Part model, mm, in its own coordinate system. A direction names the side the tool comes from. Round coordinates to 2 decimals unless told otherwise and drop trailing zeros. Loops run counter-clockwise (first coordinate to the right, second up) from the corner with the lowest first, then second, coordinate; pieces in that order, holes last. Notation, with made-up numbers: M -21.5,45 L 30.5,45 A23 ccw 30.5,63 Z; hole C -5.75,6 d2. An arc over 180 degrees is marked long. Answer as CSV lines item,"result". Start each with the question number.
Item 1: Wall check: line 1 (Y direction, x = 25.85, z = 1); line 2 (X direction, y = 2, z = 0.5); line 3 (X direction, y = 3, z = 1.25). Give the ranges that are in metal, low to high.
Item 2: Band-saw the part on C-C (z = 0.75). Give the cut face in (x, y).
Item 3: Drop flat-ended pins along their axis: pin 1 Ø4 at (x, z) = (13.5, -4) entering from -Y; pin 2 Ø3.5 at (x, y) = (18.5, 6) entering from +Z; pin 3 Ø1.5 at (x, y) = (19, 25.5) entering from +Z; pin 4 Ø1.5 at (y, z) = (17.5, -2) entering from +X. Give the stop position or say it passes through.
Item 4: Mould opens along Y. For faces 4 (the flat face through (10, 27, -4)), 5 (the cylindrical face through (24.85, 25.89, 0.76)), 6 (the flat face through (15, 25.5, -4)) say: pulls with the +Y half, pulls with the -Y half, needs draft (parallel to the pull), parting line crosses it, or undercut.
Item 5: Band-saw the part on B-B (x = 25.85). Give the cut face in (y, z), and give its area (3 significant figures).
Item 6: Band-saw the part on A-A (y = 2.15). Give the cut face in (x, z), and give its area (3 significant figures).
Item 7: Which spindle directions (+Z, -Z, +X, -X, +Y, -Y) get a long thin tool onto all of the face, cutting with end or side? Do faces 1 (the flat face through (9.287, 2, 2)), 2 (the flat face through (15, 2, 3)), 3 (the flat face through (20, 27, -4)). Say none if no direction does.
Item 8: Band-saw the part on D-D (x = 7.5). Give the cut face in (y, z).
```python
from build123d import *

# Parameters (mm, degrees)
SKETCH_1_W          = 28
SKETCH_1_H          = 28
EXTRUDE_3_DEPTH     = 1.5
SKETCH_3_W          = 28
SKETCH_3_H          = 19.5
EXTRUDE_4_DEPTH     = 2
SKETCH_5_W          = 28
SKETCH_5_H          = 15
EXTRUDE_5_DEPTH     = 0.5
SKETCH_6_W          = 11
SKETCH_6_H          = 2.266421477
EXTRUDE_6_DEPTH     = 1.5
SKETCH_7_R          = 1
CUT_EXTRUDE_4_DEPTH = 1.5
SKETCH_10_W         = 10
SKETCH_10_H         = 2.5
EXTRUDE_8_DEPTH     = 8


with BuildPart() as part:
    # Эскиз1 → Бобышка-Вытянуть3 (new body)
    with BuildSketch(Plane.XY):
        with Locations((14, 14)):
            Rectangle(SKETCH_1_W, SKETCH_1_H)
    extrude(amount=EXTRUDE_3_DEPTH)

    # Эскиз3 → Бобышка-Вытянуть4 (add)
    with BuildSketch(Plane.XY.offset(1.5)):
        with Locations((14, 13.25)):
            Rectangle(SKETCH_3_W, SKETCH_3_H)
    extrude(amount=EXTRUDE_4_DEPTH)

    # Эскиз5 → Бобышка-Вытянуть5 (add)
    with BuildSketch(Plane.XY.offset(3.5)):
        with Locations((14, 15.5)):
            Rectangle(SKETCH_5_W, SKETCH_5_H)
    extrude(amount=EXTRUDE_5_DEPTH)

    # Эскиз6 → Бобышка-Вытянуть6 (add)
    with BuildSketch(Plane.XY.offset(1.5)):
        with Locations((14.787482479, 2.366789262)):
            Rectangle(SKETCH_6_W, SKETCH_6_H)
    extrude(amount=EXTRUDE_6_DEPTH)

    # Эскиз7 → Вырез-Вытянуть4 (cut)
    with BuildSketch(Plane.XY.offset(1.5)):
        with Locations((2.15, 2.15)):
            Circle(SKETCH_7_R)
        with Locations((2.15, 25.85)):
            Circle(SKETCH_7_R)
        with Locations((25.85, 25.85)):
            Circle(SKETCH_7_R)
        with Locations((25.85, 2.15)):
            Circle(SKETCH_7_R)
    extrude(amount=-CUT_EXTRUDE_4_DEPTH, mode=Mode.SUBTRACT)

    # Эскиз10 → Бобышка-Вытянуть8 (add)
    with BuildSketch(Plane(origin=(0, 0, 0), x_dir=(-1, 0, 0), z_dir=(0, 0, -1))):
        with Locations((-15, 26.75)):
            Rectangle(SKETCH_10_W, SKETCH_10_H)
    extrude(amount=EXTRUDE_8_DEPTH)


solid = part.part
```
Answer block:
1,line 1,"y = 0 to 1.15, 3.15 to 24.85, 26.85 to 28"
1,line 2,"x = 0 to 1.16, 3.14 to 24.86, 26.84 to 28"
1,line 3,"x = 0 to 1.62, 2.68 to 25.32, 26.38 to 28"
2,outline,"M 0,0 L 28,0 L 28,28 L 0,28 Z; hole C 2.15,2.15 d2; hole C 2.15,25.85 d2; hole C 25.85,2.15 d2; hole C 25.85,25.85 d2"
3,pin 1,"stops at y = 25.5"
3,pin 2,"stops at z = 3.5"
3,pin 3,"stops at z = 1.5"
3,pin 4,"passes through"
4,face 4,"needs draft"
4,face 5,"undercut"
4,face 6,"pulls with the -Y half"
5,outline,"M 0,0 L 1.15,0 L 1.15,1.5 L 0,1.5 Z; M 3.15,0 L 24.85,0 L 24.85,1.5 L 23,1.5 L 23,4 L 8,4 L 8,3.5 L 3.5,3.5 L 3.5,1.5 L 3.15,1.5 Z; M 26.85,0 L 28,0 L 28,1.5 L 26.85,1.5 Z"
5,area,"82.5 mm^2"
6,outline,"M 0,0 L 1.15,0 L 1.15,1.5 L 0,1.5 Z; M 3.15,0 L 24.85,0 L 24.85,1.5 L 20.29,1.5 L 20.29,3 L 9.29,3 L 9.29,1.5 L 3.15,1.5 Z; M 26.85,0 L 28,0 L 28,1.5 L 26.85,1.5 Z"
6,area,"52.5 mm^2"
7,face 1,"+Z, -X, -Y"
7,face 2,"+Z, +X, -X, -Y"
7,face 3,"-Z, +X, +Y, -Y"
8,outline,"M 0,0 L 28,0 L 28,1.5 L 23,1.5 L 23,4 L 8,4 L 8,3.5 L 3.5,3.5 L 3.5,1.5 L 0,1.5 Z"
